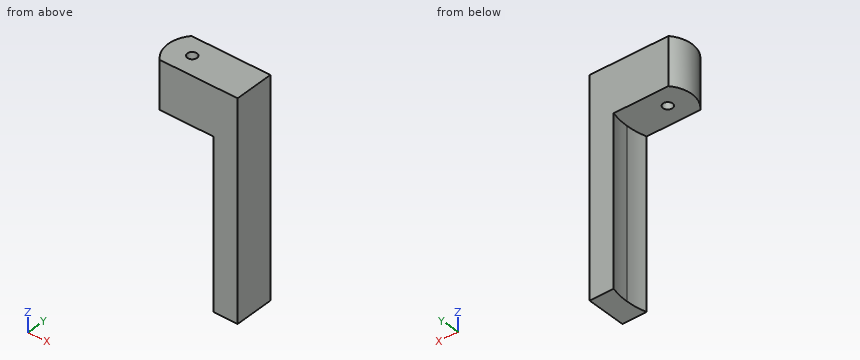
from build123d import *

# Parameters (mm, degrees)
F1_DEPTH = 35
F2_R     = 1
F3_DEPTH = 10


# Not quite as in the source:
# - a feature names something its author has since deleted; it is built from what else it names


with BuildPart() as f1:
    # F0 (on Top) → F1 (new body)
    with BuildSketch(Plane.XY):
        with BuildLine():
            ThreePointArc((-21.369307128, 4.0069422022), (-20.961114092, 2.0219241613), (-20.8242168194, 0))
            ThreePointArc((-20.8242168194, 0), (-20.9750189274, -2.1216319103), (-21.4243930811, -4.2006042786))
            Line((-21.4243930811, -4.2006042786), (-16.3557600736, -4.2006042786))
            Line((-16.3557600736, -4.2006042786), (-16.3557600736, 4.0069422022))
            Line((-16.3557600736, 4.0069422022), (-21.369307128, 4.0069422022))
        make_face()
    extrude(amount=F1_DEPTH)

    # F2 (on face) → F3 (join)
    with BuildSketch(Plane.XY.offset(35)):
        with BuildLine():
            Line((-16.3557600736, -4.2006042786), (-16.3557600736, 4.0069422022))
            Line((-16.3557600736, 4.0069422022), (-21.369307128, 4.0069422022))
            ThreePointArc((-21.369307128, 4.0069422022), (-20.8245546521, -0.1006720692), (-21.4243930811, -4.2006042786))
            Line((-21.4243930811, -4.2006042786), (-16.3557600736, -4.2006042786))
        make_face()
        with BuildLine():
            ThreePointArc((-21.4243930811, -4.2006042786), (-20.8245546521, -0.1006720692), (-21.369307128, 4.0069422022))
            Line((-21.369307128, 4.0069422022), (-32.7901337676, 4.0069422022))
            ThreePointArc((-32.7901337676, 4.0069422022), (-34.3227478364, -0.1327615841), (-32.6084814815, -4.2006042786))
            Line((-32.6084814815, -4.2006042786), (-21.4243930811, -4.2006042786))
        make_face()
        with Locations((-29.3242168194, 0)):
            Circle(F2_R, mode=Mode.SUBTRACT)
    extrude(amount=F3_DEPTH)


solid = f1.part
CAD build for the part. Positions are in the model's coordinates, mm. Coordinates: 2 decimals unless noted, no trailing zeros. Order: outer loops, then holes, each group sorted by start corner. A loop starts at its lowest first (then second) coordinate and runs counter-clockwise, first axis right, second up.
Item 1: Band-saw the part on C-C on z = 39. List the corners of the cut face in (x, y), plus the area to 3 significant figures.
Check sheet entries:
outline: (-32.79, 4.01) arc R6 ccw to (-32.61, -4.2) - (-16.36, -4.2) - (-16.36, 4.01) - close; hole circle Ø2 at (-29.32, 0)
area: 140 mm2
Item 2: Drill centre lines: L1, parallel to Z at x = -31.75, y = -1.5; L2, parallel to X at y = 0.25, z = 14; L3, parallel to X at y = 1.25, z = 10.5. Where is each one in solid material? Low to high.
Check sheet entries:
L1: z = 35 to 45
L2: x = -20.83 to -16.36
L3: x = -20.88 to -16.36
Item 3: Band-saw the part on A-A on z = 18.5. List the corners of the cut face in (x, y).
Check sheet entries:
outline: (-21.42, -4.2) - (-16.36, -4.2) - (-16.36, 4.01) - (-21.37, 4.01) arc R15 cw to start
Item 4: Band-saw the part on D-D on y = -2.25. List the corners of the cut face in (x, z), plus the area to 3 significant figures.
Check sheet entries:
outline: (-33.89, 35) - (-20.99, 35) - (-20.99, 0) - (-16.36, 0) - (-16.36, 45) - (-33.89, 45) - close
area: 338 mm2
Item 5: Band-saw the part on B-B on y = 0.5. List the corners of the cut face in (x, z).
Check sheet entries:
outline: (-34.3, 35) - (-30.19, 35) - (-30.19, 45) - (-34.3, 45) - close; (-28.46, 35) - (-20.83, 35) - (-20.83, 0) - (-16.36, 0) - (-16.36, 45) - (-28.46, 45) - close
Item 6: Pin check, flat tips, straight feed: pin 1 Ø4 at (y, z) = (0, 29) entering from -X; pin 2 Ø1 at (y, z) = (1, 32.5) entering from -X; pin 3 Ø1.5 at (x, y) = (-24, 2) entering from -Z. Stop position of each tip, or through.
Check sheet entries:
pin 1: stops at x = -20.96
pin 2: stops at x = -20.9
pin 3: stops at z = 35
